Design review of the part built by this model. Coordinates are the model's own, in mm. Face numbers are marked on the shaded views. Give positions to 0.01 mm unless a question says otherwise; leave off trailing zeros. Write each loop counter-clockwise with the first axis right and the second up, starting at its lowest first coordinate (ties: lowest second). Pieces come first, ordered by that corner, then holes. Notation, with made-up numbers: (10.25, 2.5) -> (34.25, 2.5) arc R35 ccw to (34.25, 40.5) -> close; hole circle Ø1 at (37, 55.25). An arc over 180 degrees is marked (long way). Use CSV: the item, a comma, the result in double quotes.
Autodesk Inventor part; units mm, degrees
ref_plane "YZ Plane" through (0, 0, 0) normal (1, 0, 0) x (0, 1, 0)
ref_plane "XZ Plane" through (0, 0, 0) normal (0, 1, 0) x (-1, 0, 0)
ref_plane "XY Plane" through (0, 0, 0) normal (0, 0, 1) x (1, 0, 0)
sketch "Sketch1" plane through (0, 0, 0) normal (0, 0, 1) x (1, 0, 0)
  circle A0 centre (0, 0) radius 10
  circle A1 centre (0, 0) radius 11
  dimension "d0" = 22
  dimension "d4" = 20
extrude "Extrusion1" add sketch "Sketch1" along normal blind 10
sketch "Sketch2" plane through (0, 0, 0) normal (0, 0, -1) x (-1, 0, 0)
  circle A0 centre (0, 0) radius 10
extrude "Extrusion2" add sketch "Sketch2" against normal blind 3
sketch "Sketch3" plane through (0, 0, 0) normal (0, 0, -1) x (-1, 0, 0)
  point P0 (0, 0)
  point P1 (0, 0)
hole "Hole1" at (0, 0, 0) direction (0, 0, 1) diameter 3 end through all
thread "Thread1"
fillet "Fillet1" radius 2 1 edges at (-11, 0, 0)
properties part number "Cathode Screen" material "Stainless Steel"
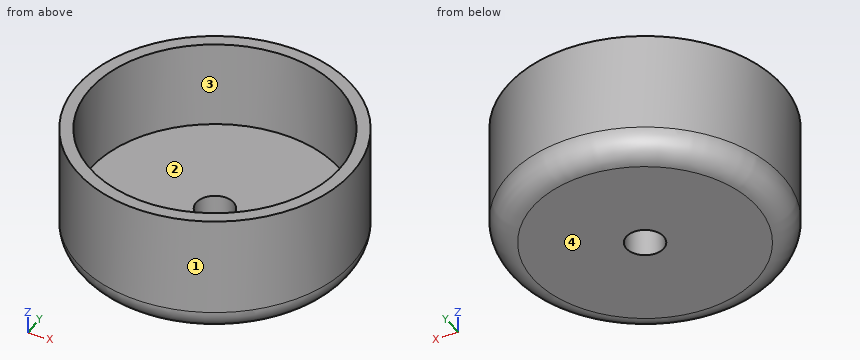
(1) Clearance check with flat-ended pins moving along their axes: pin 1 (1.5 mm diameter, centred on y = 7.5, z = 3, fed in from +X); pin 2 (10 mm diameter, centred on x = 3, y = -1, fed in from +Z); pin 3 (1.5 mm diameter, centred on y = 1.5, z = 1.5, fed in from +X). State where each tip first meets the part, or that it passes through.
Established:
pin 1,"stops at x = 8.69"
pin 2,"stops at z = 3"
pin 3,"stops at x = 10.96"
(2) Take a section at C-C (z = 7). Write out the cut boundary in (x, y), then the cut area to 3 significant figures.
Established:
outline,"circle Ø22 at (0, 0); hole circle Ø20 at (0, 0)"
area,"66.0 mm2"
(3) For line 1 along Y through (x, z) = (0, 7.25); line 2 along Z through (x, y) = (-3.75, 5); line 3 along Y through (x, z) = (3.5, 4.5), list the stretches that pass through material, from the lowest coordinate up. Write a range as [from, to].
Established:
line 1,"y = [-11, -10], [10, 11]"
line 2,"z = [0, 3]"
line 3,"y = [-10.43, -9.37], [9.37, 10.43]"
(4) Take a section at A-A (x = 0). Write out the cut boundary in (y, z).
Established:
outline,"(-11, 2) arc R2 ccw to (-9, 0) -> (-1.5, 0) -> (-1.5, 3) -> (-10, 3) -> (-10, 10) -> (-11, 10) -> close; (1.5, 0) -> (9, 0) arc R2 ccw to (11, 2) -> (11, 10) -> (10, 10) -> (10, 3) -> (1.5, 3) -> close"
(5) Mouldability with a two-part tool opening along Y and no side actions: class the marked faces 1, 2, 3 and 4 as +Y half, -Y half, draft (parallel to the pull), parting line (faces both ways), or undercut.
Established:
face 1,"parting line"
face 2,"undercut"
face 3,"undercut"
face 4,"draft"
